Geometry check sheet. Reference: the model listing, model coordinates, mm. Face numbers are marked on the shaded views. Give positions to 0.01 mm unless a question says otherwise; leave off trailing zeros. Order: outer loops, then holes, each group sorted by start corner. A loop starts at its lowest first (then second) coordinate and runs counter-clockwise, first axis right, second up.
```python
from build123d import *

# Parameters (mm, degrees)
F0_R     = 13.0048
F1_DEPTH = 20.0025
F2_DEPTH = 5.9944
F0_R_2   = 5.9944
F3_DEPTH = 13.0048


with BuildPart() as f1:
    # F0 (on Front) → F1 (new body, symmetric)
    with BuildSketch(Plane.XZ):
        with BuildLine():
            ThreePointArc((-12.949346, -21.392276), (12.278025, -21.784516), (25.0063, 0))
            ThreePointArc((25.0063, 0), (13.562501, 21.008894), (-10.294693, 22.788908))
            ThreePointArc((-10.294693, 22.788908), (-24.961282, 1.499814), (-12.949346, -21.392276))
        make_face()
        Circle(F0_R, mode=Mode.SUBTRACT)
    extrude(amount=F1_DEPTH, both=True)

    # F0 (on Front) → F2 (join, symmetric)
    with BuildSketch(Plane.XZ):
        with BuildLine():
            ThreePointArc((-12.949346, -21.392276), (-24.961282, 1.499814), (-10.294693, 22.788908))
            Line((-10.294693, 22.788908), (-102.934025, -19.060113))
            ThreePointArc((-102.934025, -19.060113), (-91.484026, -19.914411), (-85.9917, -29.9974))
            ThreePointArc((-85.9917, -29.9974), (-97.9932, -41.9989), (-109.9947, -29.9974))
            Line((-109.9947, -29.9974), (-109.9947, -70.0024))
            ThreePointArc((-109.9947, -70.0024), (-97.9932, -58.0009), (-85.9917, -70.0024))
            ThreePointArc((-85.9917, -70.0024), (-87.06104, -74.95456), (-90.078504, -79.024239))
            Line((-90.078504, -79.024239), (-23.216794, -20.367672))
            ThreePointArc((-23.216794, -20.367672), (-17.9672, -19.718852), (-12.949346, -21.392276))
        make_face()
    extrude(amount=F2_DEPTH, both=True)

    # F0 (on Front) → F3 (join, symmetric)
    with BuildSketch(Plane.XZ):
        with BuildLine():
            ThreePointArc((-85.9917, -29.9974), (-91.484026, -19.914411), (-102.934025, -19.060113))
            ThreePointArc((-102.934025, -19.060113), (-108.076189, -23.488226), (-109.9947, -29.9974))
            ThreePointArc((-109.9947, -29.9974), (-97.9932, -41.9989), (-85.9917, -29.9974))
        make_face()
        with Locations((-97.9932, -29.9974)):
            Circle(F0_R_2, mode=Mode.SUBTRACT)
        with BuildLine():
            ThreePointArc((-109.9947, -70.0024), (-102.94536, -80.93456), (-90.078504, -79.024239))
            ThreePointArc((-90.078504, -79.024239), (-87.06104, -74.95456), (-85.9917, -70.0024))
            ThreePointArc((-85.9917, -70.0024), (-97.9932, -58.0009), (-109.9947, -70.0024))
        make_face()
        with Locations((-97.9932, -70.0024)):
            Circle(F0_R_2, mode=Mode.SUBTRACT)
    extrude(amount=F3_DEPTH, both=True)


solid = f1.part
```
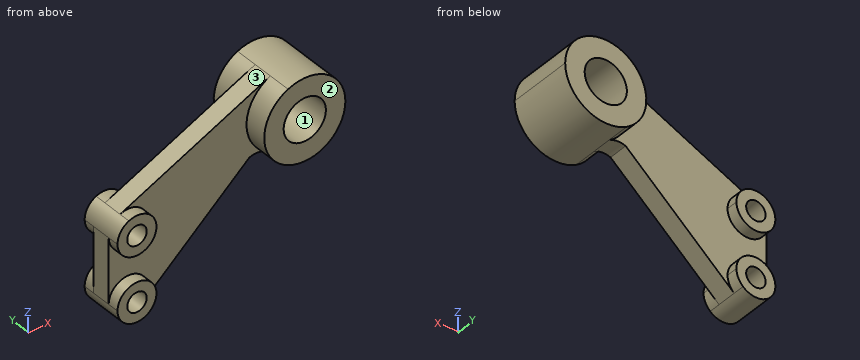
Q1. Cross-section at B-B, the plane y = 1. Record the boundary of the cut face in (x, z).
Q2. Gauge pin test, flat ends, axial feed: P1, Ø5, axis at x = -92, y = 11.5, coming from the +Z side; P2, Ø7, axis at x = -102, z = -35.5, coming from the +Y side; P3, Ø3, axis at x = -31.5, y = 0, coming from the +Z side. Record the tip position at first contact, or that the pin passes through.
Q3. Cross-section at D-D, the plane x = -99.5. Record the boundary of the cut face in (y, z).
Q4. Thickness scan on L1, parallel to Z at x = 0, y = 6; L2, parallel to Z at x = -96.5, y = -8; L3, parallel to Z at x = -101, y = 1.5. Record the ranges inside material, lowest first.
Q5. Cross-section at A-A, the plane x = 0. Record the boundary of the cut face in (y, z), and give its area (3 significant figures).
Q6. Cross-section at C-C, the plane z = -11. Record the boundary of the cut face in (x, y).
Q7. Release check for a two-part mould opening along X. For the marked faces 1, 2 and 3 record: pulls with the +X half, pulls with the -X half, needs draft (parallel to the pull), parting line crosses it, or undercut.
Answers follow:
1. outline: (-109.99, -70) arc R12 ccw to (-90.08, -79.02) - (-23.22, -20.37) arc R11.99 cw to (-12.95, -21.39) arc R25.01 ccw (long way) to (-10.29, 22.79) - (-102.93, -19.06) arc R12 ccw to (-109.99, -30) - close; hole circle Ø11.99 at (-97.99, -70); hole circle Ø11.99 at (-97.99, -30); hole circle Ø26.01 at (0, 0)
2. P1: stops at z = -18.52
2. P2: stops at y = 13
2. P3: stops at z = 13.89
3. outline: (-13, -81.91) - (13, -81.91) - (13, -75.8) - (-13, -75.8) - close; (-13, -64.2) - (13, -64.2) - (13, -58.1) - (5.99, -58.1) - (5.99, -41.9) - (13, -41.9) - (13, -35.8) - (-13, -35.8) - (-13, -41.9) - (-5.99, -41.9) - (-5.99, -58.1) - (-13, -58.1) - close; (-13, -24.2) - (13, -24.2) - (13, -18.09) - (5.99, -18.09) - (5.99, -17.51) - (-5.99, -17.51) - (-5.99, -18.09) - (-13, -18.09) - close
4. L1: z = -25.01 to -13, 13 to 25.01
4. L2: z = -81.91 to -75.81, -64.2 to -58.09, -41.91 to -35.8, -24.19 to -18.09
4. L3: z = -81.62 to -75.19, -64.82 to -35.18, -24.81 to -18.19
5. outline: (-20, -25.01) - (20, -25.01) - (20, -13) - (-20, -13) - close; (-20, 13) - (20, 13) - (20, 25.01) - (-20, 25.01) - close
5. area: 960 mm2
6. outline: (-85.09, -5.99) - (-22.46, -5.99) - (-22.46, -20) - (-6.94, -20) - (-6.94, 20) - (-22.46, 20) - (-22.46, 5.99) - (-85.09, 5.99) - close; (6.94, -20) - (22.46, -20) - (22.46, 20) - (6.94, 20) - close
7. face 1: undercut
7. face 2: needs draft
7. face 3: pulls with the -X half
